Could you check a few things on this model? Use its own coordinates, in mm. A direction names the side the tool comes from. Coordinates: 2 decimals unless noted, no trailing zeros. Order: outer loops, then holes, each group sorted by start corner. A loop starts at its lowest first (then second) coordinate and runs counter-clockwise, first axis right, second up. Notation, with made-up numbers: (70, 27) -> (80, 27) arc R23 ccw to (80, 52) -> close; hole circle Ø3 at (12.25, -36.75). An arc over 180 degrees is marked (long way). Use a Markdown table: item, result. Add a question column.
1) If I drill on L1, parallel to Y at x = -12.75, z = 0; L2, parallel to X at y = -4.5, z = 13; L3, parallel to X at y = 25.5, z = 38.5, over which ranges is the centre line in solid material (lowest first)? Write a range as [from, to].
2) Will these pins go through, and if not, where does the flat tip stop? pin 1 Ø3 at (x, y) = (-40, -36.5) entering from -Z; pin 2 Ø5 at (y, z) = (-44.5, 0) entering from -X; pin 3 Ø3.5 at (y, z) = (-31, 31) entering from +X.
3) Thinking about a two-plate mould opening in Z: for faces 3 (the flat face through (-53.7, -5, 27)), 4 (the flat face through (-50.7, 0, 0)), which applies, +Z half, -Z half, draft (parallel to the pull), parting line (faces both ways), or undercut?
4) If we section it at B-B (x = -17.5): Write out the boundary of the cut face in (y, z), plus the area to 3 significant figures.
5) If we section it at A-A (x = -11): Give the number of separate pieces and of enclosed holes in the cut face, plus the area to 3 significant figures.
6) Which directions (+Z, -Z, +X, -X, +Y, -Y) give clear straight access to the entire face, cutting with the end or side of a thin tool? Please do faces 1 (the flat face through (-46.7, -39, 16)), 2 (the flat face through (-16, 31, 31)).
```python
from build123d import *

# Parameters (mm, degrees)
SKETCH1_W                         = 42.7
SKETCH1_H                         = 49
SKETCH2_R                         = 35.5
BOSS_EXTRUDE1_DEPTH               = 11.2
CUT_EXTRUDE1_START                = -8
CUT_EXTRUDE1_DEPTH                = 8
SKETCH4_R                         = 40
BOSS_EXTRUDE2_DEPTH               = 3
SKETCH5_R                         = 40
BOSS_EXTRUDE3_DEPTH               = 4
BOSS_EXTRUDE3_TAPER               = 45.000000001
M33_CLEARANCE_HOLE1_D             = 35.4
M33_CLEARANCE_HOLE1_DEPTH         = 7.5
SKETCH8_W                         = 8.5
SKETCH8_H                         = 17.5
F_3_0_3_DIAMETER_HOLE1_D          = 3
F_3_0_3_DIAMETER_HOLE1_DEPTH      = 4
F_3_0_3_DIAMETER_HOLE2_D          = 3
F_3_0_3_DIAMETER_HOLE2_DEPTH      = 8
F_21_0_21_DIAMETER_HOLE1_D        = 21
F_21_0_21_DIAMETER_HOLE1_DEPTH    = 4.5
F_4_0_4_DIAMETER_HOLE1_D          = 4
F_4_0_4_DIAMETER_HOLE1_DEPTH      = 8
F_3_0_3_DIAMETER_HOLE3_D          = 3
F_3_0_3_DIAMETER_HOLE3_DEPTH      = 3
CHAMFER1_SIZE                     = 0.5
SKETCH19_R                        = 38.44010433
CUT_EXTRUDE2_DEPTH                = 10.2
CUT_EXTRUDE3_START                = -1
SKETCH20_R                        = 38.36803995
SKETCH20_R_2                      = 35.5
SKETCH20_R_3                      = 34
SKETCH20_R_4                      = 32.5
CUT_EXTRUDE3_DEPTH                = 1
TAP_DRILL_FOR_M3_TAP2_D           = 2.5
TAP_DRILL_FOR_M3_TAP2_DEPTH       = 2
TAP_DRILL_FOR_M3_TAP2_CSINK_D     = 2.55
TAP_DRILL_FOR_M3_TAP2_CSINK_ANGLE = 90
TAP_DRILL_FOR_M3_TAP2_TIP         = 0.751075774
SKETCH24_R                        = 2.55
SKETCH24_R_2                      = 1.25
BOSS_EXTRUDE4_DEPTH               = 3


with BuildPart() as part:
    # Sketch1 → Revolve1 (revolve)
    with BuildSketch(Plane.XY, mode=Mode.PRIVATE) as revolve1_sk:
        with Locations((-29.35, 24.5)):
            Rectangle(SKETCH1_W, SKETCH1_H)
    revolve(revolve1_sk.sketch.rotate(Axis((-50.7, 0, 0), (1, 0, 0)), 270), axis=Axis((-50.7, 0, 0), (1, 0, 0)))

    # Sketch2 → Boss-Extrude1 (add)
    with BuildSketch(Plane.ZY.offset(50.7)):
        Circle(SKETCH2_R)
    extrude(amount=BOSS_EXTRUDE1_DEPTH)

    # Sketch3 → Cut-Extrude1 (cut)
    with BuildSketch(Plane.ZY.offset(61.9).offset(CUT_EXTRUDE1_START)):
        with BuildLine():
            Line((5.253044864, 35.109194233), (32.553289394, 14.160979826))
            ThreePointArc((32.553289394, 14.160979826), (21.61103073, 28.16404358), (5.253044864, 35.109194233))
        make_face()
    extrude(amount=CUT_EXTRUDE1_DEPTH, mode=Mode.SUBTRACT)

    # Sketch4 → Boss-Extrude2 (add)
    with BuildSketch(Plane(origin=(-8, 0, 0), x_dir=(0, 0, -1), z_dir=(1, 0, 0))):
        Circle(SKETCH4_R)
    extrude(amount=BOSS_EXTRUDE2_DEPTH)

    # Sketch5 → Boss-Extrude3 (add)
    with BuildSketch(Plane(origin=(-5, 0, 0), x_dir=(0, 0, -1), z_dir=(1, 0, 0))):
        Circle(SKETCH5_R)
    extrude(amount=BOSS_EXTRUDE3_DEPTH, taper=BOSS_EXTRUDE3_TAPER)

    # M33 Clearance Hole1
    with Locations(Plane(origin=(-1, 0, 0), x_dir=(0, 0, -1), z_dir=(1, 0, 0))):
        with Locations((0, 0)):
            Hole(M33_CLEARANCE_HOLE1_D / 2, depth=M33_CLEARANCE_HOLE1_DEPTH)

    # Sketch8 → Revolve2 (revolve)
    with BuildSketch(Plane.XY, mode=Mode.PRIVATE) as revolve2_sk:
        with Locations((-4.25, 8.75)):
            Rectangle(SKETCH8_W, SKETCH8_H)
    revolve(revolve2_sk.sketch.rotate(Axis((-8.5, 0, 0), (1, 0, 0)), 270), axis=Axis((-8.5, 0, 0), (1, 0, 0)))

    # Ø3.0 (3) Diameter Hole1
    with Locations(Plane.ZY.offset(50.7)):
        with Locations((39.264880132, 16.264045876), (39.264880132, -16.264045876), (16.264045876, -39.264880132), (-16.264045876, -39.264880132), (-39.264880132, -16.264045876), (-39.264880132, 16.264045876), (-16.264045876, 39.264880132), (16.264045876, 39.264880132)):
            Hole(F_3_0_3_DIAMETER_HOLE1_D / 2, depth=F_3_0_3_DIAMETER_HOLE1_DEPTH)

    # Ø3.0 (3) Diameter Hole2
    with Locations(Plane(origin=(-8, 0, 0), x_dir=(0, 0, -1), z_dir=(1, 0, 0))):
        with Locations((31.466251763, 31.466251763), (44.5, 0), (31.466251763, -31.466251763), (0, -44.5), (-31.466251763, -31.466251763), (-44.5, 0), (-31.466251763, 31.466251763), (0, 44.5)):
            Hole(F_3_0_3_DIAMETER_HOLE2_D / 2, depth=F_3_0_3_DIAMETER_HOLE2_DEPTH)

    # Ø21.0 (21) Diameter Hole1
    with Locations(Plane(origin=(0, 0, 0), x_dir=(0, 0, -1), z_dir=(1, 0, 0))):
        with Locations((0, 0)):
            Hole(F_21_0_21_DIAMETER_HOLE1_D / 2, depth=F_21_0_21_DIAMETER_HOLE1_DEPTH)

    # Ø4.0 (4) Diameter Hole1
    with Locations(Plane(origin=(0, 0, 0), x_dir=(0, 0, -1), z_dir=(1, 0, 0))):
        with Locations((-14, 0), (-7, 12.124355653), (7, 12.124355653), (14, 0), (7, -12.124355653), (-7, -12.124355653)):
            Hole(F_4_0_4_DIAMETER_HOLE1_D / 2, depth=F_4_0_4_DIAMETER_HOLE1_DEPTH)

    # Ø3.0 (3) Diameter Hole3
    with Locations(Plane(origin=(0, 0, 0), x_dir=(0, 0, -1), z_dir=(1, 0, 0))):
        with Locations((0, -14), (0, 14)):
            Hole(F_3_0_3_DIAMETER_HOLE3_D / 2, depth=F_3_0_3_DIAMETER_HOLE3_DEPTH)

    # Chamfer1
    chamfer1_edges = [part.edges().sort_by_distance(p)[0] for p in [
        (0, 0, 17.5),
        (-8, 0, 49),
        (-50.7, 0, 49),
    ]]
    chamfer(chamfer1_edges, length=CHAMFER1_SIZE)

    # Sketch19 → Cut-Extrude2 (cut)
    with BuildSketch(Plane.ZY.offset(61.9)):
        Circle(SKETCH19_R)
    extrude(amount=-CUT_EXTRUDE2_DEPTH, mode=Mode.SUBTRACT)

    # Sketch20 → Cut-Extrude3 (cut)
    # profile 1 of 3: a face of its own
    with BuildSketch(Plane.ZY.offset(51.7).offset(CUT_EXTRUDE3_START)):
        Circle(SKETCH20_R)
        Circle(SKETCH20_R_2, mode=Mode.SUBTRACT)
    # profile 2 of 3: a face of its own
    with BuildSketch(Plane.ZY.offset(51.7).offset(CUT_EXTRUDE3_START)):
        Circle(SKETCH20_R_2)
        Circle(SKETCH20_R_3, mode=Mode.SUBTRACT)
    # profile 3 of 3: a face of its own
    with BuildSketch(Plane.ZY.offset(51.7).offset(CUT_EXTRUDE3_START)):
        Circle(SKETCH20_R_4)
    extrude(amount=CUT_EXTRUDE3_DEPTH, mode=Mode.SUBTRACT)

    # Tap Drill for M3 Tap2
    with Locations(Plane.ZY.offset(50.7)):
        with Locations((-16.740939298, -21.817216858), (-10.52379439, 25.406687144), (27.264733688, -3.589470286)):
            CounterSinkHole(TAP_DRILL_FOR_M3_TAP2_D / 2, TAP_DRILL_FOR_M3_TAP2_CSINK_D / 2, depth=TAP_DRILL_FOR_M3_TAP2_DEPTH, counter_sink_angle=TAP_DRILL_FOR_M3_TAP2_CSINK_ANGLE)
            with Locations((0, 0, -(TAP_DRILL_FOR_M3_TAP2_DEPTH + TAP_DRILL_FOR_M3_TAP2_TIP / 2))):  # 118° drill point
                Cone(0, TAP_DRILL_FOR_M3_TAP2_D / 2, TAP_DRILL_FOR_M3_TAP2_TIP, mode=Mode.SUBTRACT)

    # Sketch24 → Boss-Extrude4 (add)
    # profile 1 of 3: a face of its own
    with BuildSketch(Plane.ZY.offset(50.7)):
        with Locations((-10.52379439, 25.406687144)):
            Circle(SKETCH24_R)
        with Locations((-10.52379439, 25.406687144)):
            Circle(SKETCH24_R_2, mode=Mode.SUBTRACT)
    # profile 2 of 3: a face of its own
    with BuildSketch(Plane.ZY.offset(50.7)):
        with Locations((-16.740939298, -21.817216858)):
            Circle(SKETCH24_R)
        with Locations((-16.740939298, -21.817216858)):
            Circle(SKETCH24_R_2, mode=Mode.SUBTRACT)
    # profile 3 of 3: a face of its own
    with BuildSketch(Plane.ZY.offset(50.7)):
        with Locations((27.264733688, -3.589470286)):
            Circle(SKETCH24_R)
        with Locations((27.264733688, -3.589470286)):
            Circle(SKETCH24_R_2, mode=Mode.SUBTRACT)
    extrude(amount=BOSS_EXTRUDE4_DEPTH)


solid = part.part
```
Answer sheet:
| question | item | result |
|---|---|---|
| 1 | L1 | [-49, -46], [-43, 43], [46, 49] |
| 1 | L2 | [-50.7, 0] |
| 1 | L3 | [-50.7, -8] |
| 2 | pin 1 | z = -34.29 |
| 2 | pin 2 | x = -50.7 |
| 2 | pin 3 | x = -8 |
| 3 | face 3 | draft |
| 3 | face 4 | undercut |
| 4 | outline | circle Ø98 at (0, 0) |
| 4 | area | 7,540 mm2 |
| 5 | separate pieces | 1 |
| 5 | enclosed holes | 8 |
| 5 | area | 7,490 mm2 |
| 6 | face 1 | -X |
| 6 | face 2 | +X |
